from build123d import *

# Parameters (mm, degrees)
SKETCH1_W           = 27.8
SKETCH1_H           = 28
SKETCH1_R           = 2.55
BOSS_EXTRUDE1_DEPTH = 3.5
SKETCH2_W           = 27.8
SKETCH2_H           = 15.9
SKETCH2_R           = 1.55
BOSS_EXTRUDE2_DEPTH = 3
SKETCH3_W           = 6
SKETCH3_H           = 6
CUT_EXTRUDE5_DEPTH  = 3.5
SKETCH4_W           = 6
SKETCH4_H           = 6
SKETCH4_H_2         = 1
CUT_EXTRUDE7_DEPTH  = 3.5
SKETCH5_R           = 2.55
SKETCH5_R_2         = 5
CUT_EXTRUDE8_DEPTH  = 3


with BuildPart() as part:
    # Sketch1 → Boss-Extrude1 (new body)
    with BuildSketch(Plane(origin=(0, 0, 0), x_dir=(1, 0, 0), z_dir=(0, 1, 0))):
        with Locations((13.9, 14)):
            Rectangle(SKETCH1_W, SKETCH1_H)
        with Locations(Location((13.65, 23.68, 0), (0, 0, 270))):
            Circle(SKETCH1_R, mode=Mode.SUBTRACT)
        with Locations(Location((3.65, 23.68, 0), (0, 0, 270))):
            Circle(SKETCH1_R, mode=Mode.SUBTRACT)
    extrude(amount=BOSS_EXTRUDE1_DEPTH)

    # Sketch2 → Boss-Extrude2 (add)
    with BuildSketch(Plane(origin=(0, 3.5, 0), x_dir=(1, 0, 0), z_dir=(0, 1, 0))):
        with Locations((13.9, 7.95)):
            Rectangle(SKETCH2_W, SKETCH2_H)
        with Locations(Location((2.8, 2.8, 0), (0, 0, 270))):
            Circle(SKETCH2_R, mode=Mode.SUBTRACT)
        with Locations(Location((25, 13.1, 0), (0, 0, 270))):
            Circle(SKETCH2_R, mode=Mode.SUBTRACT)
    extrude(amount=BOSS_EXTRUDE2_DEPTH)

    # Sketch3 → Cut-Extrude5 (cut)
    with BuildSketch(Plane.XZ):
        with Locations((3, -3)):
            Rectangle(SKETCH3_W, SKETCH3_H)
    extrude(amount=-CUT_EXTRUDE5_DEPTH, mode=Mode.SUBTRACT)

    # Sketch4 → Cut-Extrude7 (cut)
    with BuildSketch(Plane.XZ):
        with Locations((24.8, -12.9)):
            Rectangle(SKETCH4_W, SKETCH4_H)
        with Locations((24.8, -16.4)):
            Rectangle(SKETCH4_W, SKETCH4_H_2)
    extrude(amount=-CUT_EXTRUDE7_DEPTH, mode=Mode.SUBTRACT)

    # Sketch5 → Cut-Extrude8 (cut)
    with BuildSketch(Plane.XZ):
        with Locations(Location((13.65, -23.68, 0), (0, 0, 90))):
            Circle(SKETCH5_R)
        with Locations((23.65, -13.68)):
            Circle(SKETCH5_R_2)
    extrude(amount=-CUT_EXTRUDE8_DEPTH, mode=Mode.SUBTRACT)


solid = part.part
Geometry: final body of the model. Coordinates: model frame, mm. A direction names the side the tool comes from. Round coordinates to 2 decimals unless told otherwise and drop trailing zeros. Order: outer loops, then holes, each group sorted by start corner. A loop starts at its lowest first (then second) coordinate and runs counter-clockwise, first axis right, second up.
Q1. Section D-D, the plane z = -2. Output: boundary loops of the cut face in (x, y).
Result sheet:
outline: (0, 3.5) - (1.47, 3.5) - (1.47, 6.5) - (0, 6.5) - close; (4.13, 3.5) - (6, 3.5) - (6, 0) - (27.8, 0) - (27.8, 6.5) - (4.13, 6.5) - close
Q2. Pin query (flat end, axial travel): pin 1 (8 mm diameter, centred on x = 13.65, z = -23.68, fed in from +Y); pin 2 (5 mm diameter, centred on x = 23, z = -12.5, fed in from -Y); pin 3 (0.9 mm diameter, centred on x = 13, y = 5, fed in from -Z); pin 4 (3 mm diameter, centred on x = 25, z = -13.1, fed in from +Y). Return the tip coordinate at first contact, or that it passes through.
Result sheet:
pin 1: stops at y = 3.5
pin 2: stops at y = 3
pin 3: stops at z = -15.9
pin 4: passes through
Q3. Material intervals for probe 1 along X at (y, z) = (1.3, -23.68); probe 2 along Y at (x, z) = (26.5, -25.75); probe 3 along X at (y, z) = (1, -13.68), sorted ascending.
Result sheet:
probe 1: x = 0 to 1.1, 6.2 to 11.1, 16.2 to 27.8
probe 2: y = 0 to 3.5
probe 3: x = 0 to 18.65
Q4. Section B-B, the plane x = 13.65. Output: boundary loops of the cut face in (y, z), and give its area (3 significant figures).
Result sheet:
outline: (0, -28) - (3.5, -28) - (3.5, -26.23) - (0, -26.23) - close; (0, -21.13) - (3.5, -21.13) - (3.5, -15.9) - (6.5, -15.9) - (6.5, 0) - (0, 0) - close
area: 128 mm2
Q5. Access query for faces 5 (the face through (23, 3.5, -13)), 6 (the face through (4.3, 3.5, -3.6)), 7 (the face through (14, 3.5, -21)), 8 (the face through (18.655, 1.479, -13.908)). Directions: +Z, -Z, +X, -X, +Y, -Y. A direction counts if a zero-diameter tool reaches every point of the face in a straight line with its end or side. Return the directions, or none.
Result sheet:
face 5: +X, -Y
face 6: +Z, -X, -Y
face 7: -Z, +X, -X, +Y
face 8: -Y
Q6. Section C-C, the plane x = 3.65. Output: boundary loops of the cut face in (y, z).
Result sheet:
outline: (0, -28) - (3.5, -28) - (3.5, -26.23) - (0, -26.23) - close; (0, -21.13) - (3.5, -21.13) - (3.5, -15.9) - (6.5, -15.9) - (6.5, -4.1) - (3.5, -4.1) - (3.5, -6) - (0, -6) - close; (3.5, -1.5) - (6.5, -1.5) - (6.5, 0) - (3.5, 0) - close
Q7. Mould query, pull axis X, two halves, no side actions, for faces 1 (the face through (6, 2, -3)), 2 (the face through (12.098, 1.726, -25.704)), 3 (the face through (3.762, 1.726, -26.228)), 4 (the face through (25.2, 3.2, -16.9)). Classes: released by +X, released by -X, zero draft, split by the parting line, or undercut.
Result sheet:
face 1: released by -X
face 2: undercut
face 3: undercut
face 4: zero draft
Q8. Section A-A, the plane z = -23.68. Output: boundary loops of the cut face in (x, y), and give its area (3 significant figures).
Result sheet:
outline: (0, 0) - (1.1, 0) - (1.1, 3.5) - (0, 3.5) - close; (6.2, 0) - (11.1, 0) - (11.1, 3.5) - (6.2, 3.5) - close; (16.2, 0) - (27.8, 0) - (27.8, 3.5) - (16.2, 3.5) - close
area: 61.6 mm2
